```python
from build123d import *

# Parameters (mm, degrees)
SKETCH_1_W               = 24
SKETCH_1_H               = 24
EXTRUDE_1_DEPTH          = 24
SKETCH_2_W               = 71.732005
SKETCH_2_H               = 64.325513166
CUT_EXTRUDE_1_DEPTH      = 24
SKETCH_3_W               = 19.1
SKETCH_3_H               = 19.1
CUT_EXTRUDE_2_DEPTH      = 0.75
SKETCH_4_R               = 20.316156742
SKETCH_4_R_2             = 15
CUT_EXTRUDE_3_DEPTH      = 3
SKETCH_5_R               = 19.778815759
SKETCH_5_R_2             = 15
CUT_EXTRUDE_4_DEPTH      = 3
SKETCH_6_R               = 1.2
CUT_EXTRUDE_5_DEPTH      = 8
CUT_EXTRUDE_6_DEPTH      = 0.1
CUT_EXTRUDE_6_DEPTH_BACK = 0.1
SKETCH_7_W               = 8.073607186
SKETCH_7_H               = 16
CUT_EXTRUDE_7_DEPTH      = 15
CUT_EXTRUDE_7_DEPTH_BACK = 15


with BuildPart() as part:
    # Sketch 1 → Extrude 1 (new body)
    with BuildSketch(Plane(origin=(0, 0, 0), x_dir=(1, 0, 0), z_dir=(0, 1, 0))):
        Rectangle(SKETCH_1_W, SKETCH_1_H)
    extrude(amount=EXTRUDE_1_DEPTH)

    # Sketch 2 → Cut-Extrude 1 (cut)
    with BuildSketch(Plane(origin=(-6, 6, 0), x_dir=(0.7071067811865477, 0.7071067811865475, 0), z_dir=(-0.7071067811865475, 0.7071067811865477, 0))):
        Rectangle(SKETCH_2_W, SKETCH_2_H)
    extrude(amount=CUT_EXTRUDE_1_DEPTH, mode=Mode.SUBTRACT)

    # Sketch 3 → Cut-Extrude 2 (cut)
    with BuildSketch(Plane(origin=(-6, 6, 0), x_dir=(0.7071067811865476, 0.7071067811865476, 0), z_dir=(-0.7071067811865476, 0.7071067811865476, 0))):
        with Locations((8.485281374, 0)):
            Rectangle(SKETCH_3_W, SKETCH_3_H)
    extrude(amount=-CUT_EXTRUDE_2_DEPTH, mode=Mode.SUBTRACT)

    # Sketch 4 → Cut-Extrude 3 (cut)
    with BuildSketch(Plane.XY.offset(10)):
        with Locations((0, 12.288929334)):
            Circle(SKETCH_4_R)
        with Locations((0, 12.288929334)):
            Circle(SKETCH_4_R_2, mode=Mode.SUBTRACT)
    extrude(amount=-CUT_EXTRUDE_3_DEPTH, mode=Mode.SUBTRACT)

    # Sketch 5 → Cut-Extrude 4 (cut)
    with BuildSketch(Plane.XY.offset(-10)):
        with Locations((0, 11.885010241)):
            Circle(SKETCH_5_R)
        with Locations((0, 11.885010241)):
            Circle(SKETCH_5_R_2, mode=Mode.SUBTRACT)
    extrude(amount=CUT_EXTRUDE_4_DEPTH, mode=Mode.SUBTRACT)

    # Sketch 6 → Cut-Extrude 5 (cut)
    with BuildSketch(Plane(origin=(0, 0, 0), x_dir=(1, 0, 0), z_dir=(0, 1, 0))):
        with Locations(Location((0, 0, 0), (0, 0, 270))):
            Circle(SKETCH_6_R)
    extrude(amount=CUT_EXTRUDE_5_DEPTH, mode=Mode.SUBTRACT)

    # Sketch 7 → Cut-Extrude 6 (cut, two sides: drawn at the far end of the back side and taken through both)
    with BuildSketch(Plane(origin=(0, 0, 0), x_dir=(0, 0, -1), z_dir=(1, 0, 0)).offset(-CUT_EXTRUDE_6_DEPTH_BACK)):
        Rectangle(SKETCH_7_W, SKETCH_7_H)
    extrude(amount=CUT_EXTRUDE_6_DEPTH + CUT_EXTRUDE_6_DEPTH_BACK, mode=Mode.SUBTRACT)

    # Sketch 8 → Cut-Extrude 7 (cut, two sides: drawn at the far end of the back side and taken through both)
    with BuildSketch(Plane.XY.offset(-CUT_EXTRUDE_7_DEPTH_BACK)):
        Polygon((0.926133031, -2.090276762), (18.080980338, 21.871040762), (23.544619253, -7.469690988), align=None)
    extrude(amount=CUT_EXTRUDE_7_DEPTH + CUT_EXTRUDE_7_DEPTH_BACK, mode=Mode.SUBTRACT)


solid = part.part
```
Source: CAD feature listing. Evaluate the final solid. Frame: model axes, mm. A direction names the side the tool comes from. Coordinates: 2 decimals unless noted, no trailing zeros. Loops run counter-clockwise (first coordinate to the right, second up) from the corner with the lowest first, then second, coordinate; pieces in that order, holes last. Notation, with made-up numbers: M -36.75,28 L 12.25,28 A19 cw 12.25,60 Z; hole C 86.5,-37.5 d8. An arc over 180 degrees is marked long. Use CSV: the item, a comma, the result in double quotes.
(1) Contact query for flat-ended pins moving along their axis: pin 1 (1.4 mm diameter, centred on y = 5.5, z = -2.5, fed in from -X); pin 2 (5 mm diameter, centred on x = 8.5, z = -6.5, fed in from -Y); pin 3 (2.5 mm diameter, centred on y = 2.5, z = 3, fed in from -X); pin 4 (1 mm diameter, centred on x = 3.5, y = 18.5, fed in from +Z). Output: stop coordinate, or through.
Answers follow:
pin 1,"x = -7.2"
pin 2,"y = 5"
pin 3,"x = -10.75"
pin 4,"through"
(2) Reachability of faces 1 (the face through (11.315, 21.732, -8.521)), 2 (the face through (-9.575, 0.743, 8.521)), 3 (the face through (8, 20, 0)), 4 (the face through (-0.1, 4, -3)) from +Z, -Z, +X, -X, +Y, -Y: full face, straight path, thin tool, end or side. Return the list, or none.
Answers follow:
face 1,"+X, +Y"
face 2,"-X, -Y"
face 3,"+Z, -Z, -X, +Y"
face 4,"-Y"
(3) Draft query along X for faces 5 (the face through (0.1, 4, 3)), 6 (the face through (-10.6, 0.4, -10)), 7 (the face through (-9.94, 0.65, -8.52)), 8 (the face through (0.1, 4, -3)). Return one class per face: pulls with the +X half, pulls with the -X half, needs draft (parallel to the pull), parting line crosses it, or undercut.
Answers follow:
face 5,"undercut"
face 6,"needs draft"
face 7,"pulls with the -X half"
face 8,"undercut"
(4) Cut plane D-D on z = 7.5. Return loops of the section in (x, y).
Answers follow:
outline,"M -10.46,1.54 A15 ccw -8.6,0 L 2.42,0 L 12,13.38 L 12,21.29 A15 ccw 10.75,22.75 L 6.75,18.75 L 7.28,18.22 L -6.22,4.72 L -6.75,5.25 Z"
(5) Line query: line 1 (X direction, y = 6.5, z = -0.25); line 2 (Y direction, x = 0.5, z = -6); line 3 (X direction, y = 1.75, z = -2.25). Output: solid intervals per line, ascending. Write a range as [from, to].
Answers follow:
line 1,"[-4.44, -1.17], [1.17, 7.08]"
line 2,"[0, 11.44]"
line 3,"[-10.25, -0.1], [0.1, 3.68]"
(6) Cut plane B-B on y = 7.5. Return loops of the section in (x, z), and give its area (3 significant figures).
Answers follow:
outline,"M -4.5,-12 L 7.79,-12 L 7.79,12 L -4.5,12 L -4.5,9.55 L -3.44,9.55 L -3.44,-9.55 L -4.5,-9.55 Z; hole M -0.1,-4.04 L 0.1,-4.04 L 0.1,-1.2 A1.2 ccw 0.1,1.2 L 0.1,4.04 L -0.1,4.04 L -0.1,1.2 A1.2 ccw -0.1,-1.2 Z"
area,"269 mm²"
(7) Cut plane C-C on x = -4. Return loops of the section in (y, z), and give its area (3 significant figures).
Answers follow:
outline,"M 0,-12 L 8,-12 L 8,-9.55 L 6.94,-9.55 L 6.94,9.55 L 8,9.55 L 8,12 L 0,12 Z"
area,"172 mm²"
(8) Cut plane A-A on z = -5.75. Return loops of the section in (x, y).
Answers follow:
outline,"M -12,0 L 2.42,0 L 12,13.38 L 12,24 L 6.75,18.75 L 7.28,18.22 L -6.22,4.72 L -6.75,5.25 Z"
